```python
from build123d import *

# Parameters (mm, degrees)
SKETCH_8_R          = 1.5
SKETCH_8_W          = 15
SKETCH_8_H          = 16
EXTRUDE_4_DEPTH     = 4
SKETCH_9_R          = 7.5
EXTRUDE_5_DEPTH     = 5
SKETCH_10_R         = 5
EXTRUDE_6_DEPTH     = 5
SKETCH_12_R         = 4.5
EXTRUDE_7_DEPTH     = 1.1
SKETCH_14_R         = 1.45
CUT_EXTRUDE_1_DEPTH = 24.070760716
SKETCH_15_R         = 5
EXTRUDE_8_DEPTH     = 2
FILLET_2_R          = 0.75
SKETCH_16_R         = 1.45
CUT_EXTRUDE_2_DEPTH = 25.426624818


with BuildPart() as part:
    # 草图8 → 凸台-拉伸4 (new body)
    # profile 1 of 3: a face of its own
    with BuildSketch(Plane(origin=(0, 0, 0), x_dir=(1, 0, 0), z_dir=(0, 1, 0))):
        with BuildLine():
            Line((-7.5, 8), (-7.5, -8))
            ThreePointArc((-7.5, -8), (-15.5, 0), (-7.5, 8))
        make_face()
        with Locations(Location((-11, 0, 0), (0, 0, 270))):
            Circle(SKETCH_8_R, mode=Mode.SUBTRACT)
    # profile 2 of 3: a face of its own
    with BuildSketch(Plane(origin=(0, 0, 0), x_dir=(1, 0, 0), z_dir=(0, 1, 0))):
        Rectangle(SKETCH_8_W, SKETCH_8_H)
    # profile 3 of 3: a face of its own
    with BuildSketch(Plane(origin=(0, 0, 0), x_dir=(1, 0, 0), z_dir=(0, 1, 0))):
        with BuildLine():
            Line((7.5, 8), (7.5, -8))
            ThreePointArc((7.5, -8), (15.5, 0), (7.5, 8))
        make_face()
        with Locations(Location((11, 0, 0), (0, 0, 270))):
            Circle(SKETCH_8_R, mode=Mode.SUBTRACT)
    extrude(amount=EXTRUDE_4_DEPTH)

    # 草图9 → 凸台-拉伸5 (add)
    with BuildSketch(Plane(origin=(0, 4, 0), x_dir=(1, 0, 0), z_dir=(0, 1, 0))):
        with Locations(Location((0, 0, 0), (0, 0, 270))):
            Circle(SKETCH_9_R)
    extrude(amount=EXTRUDE_5_DEPTH)

    # 草图10 → 凸台-拉伸6 (add)
    with BuildSketch(Plane(origin=(0, 9, 0), x_dir=(1, 0, 0), z_dir=(0, 1, 0))):
        with Locations(Location((0, 0, 0), (0, 0, 270))):
            Circle(SKETCH_10_R)
    extrude(amount=EXTRUDE_6_DEPTH)

    # 草图12 → 凸台-拉伸7 (add)
    with BuildSketch(Plane(origin=(0, 14, 0), x_dir=(1, 0, 0), z_dir=(0, 1, 0))):
        with Locations(Location((0, 0, 0), (0, 0, 270))):
            Circle(SKETCH_12_R)
    extrude(amount=EXTRUDE_7_DEPTH)

    # 草图14 → 切除-拉伸1 (cut, through all)
    with BuildSketch(Plane.XZ):
        with Locations(Location((0, 0, 0), (0, 0, 270))):
            Circle(SKETCH_14_R)
    extrude(amount=-CUT_EXTRUDE_1_DEPTH, mode=Mode.SUBTRACT)

    # 草图15 → 凸台-拉伸8 (add)
    with BuildSketch(Plane(origin=(0, 15.1, 0), x_dir=(1, 0, 0), z_dir=(0, 1, 0))):
        with Locations(Location((0, 0, 0), (0, 0, 270))):
            Circle(SKETCH_15_R)
    extrude(amount=EXTRUDE_8_DEPTH)

    # 圆角2
    fillet_2_edges = [part.edges().sort_by_distance(p)[0] for p in [
        (0, 9, -7.5),
        (0, 17.1, -5),
    ]]
    fillet(fillet_2_edges, radius=FILLET_2_R)

    # 草图16 → 切除-拉伸2 (cut, through all)
    with BuildSketch(Plane(origin=(0, 0, 0), x_dir=(-1, 0, 0), z_dir=(0, -1, 0))):
        with Locations(Location((0, 0, 0), (0, 0, 90))):
            Circle(SKETCH_16_R)
    extrude(amount=-CUT_EXTRUDE_2_DEPTH, mode=Mode.SUBTRACT)


solid = part.part
```
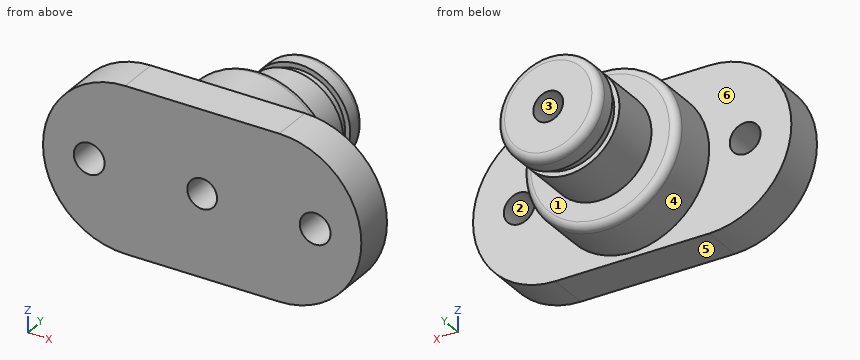
CAD build for the part. Positions are in the model's coordinates, mm. Face numbers are marked on the shaded views. A direction names the side the tool comes from. Coordinates: 2 decimals unless noted, no trailing zeros. Write each loop counter-clockwise with the first axis right and the second up, starting at its lowest first coordinate (ties: lowest second). Pieces come first, ordered by that corner, then holes. Notation, with made-up numbers: (2, 4) -> (36, 4) arc R21 ccw to (36, 25) -> close; hole circle Ø8 at (56, 27). An arc over 180 degrees is marked (long way). Return JSON: item names as keys, results as strings. Group by question number.
Q1. Pull direction Z, two halves, no side cores. Call the marked faces 1, 2, 3 and 4: released by +Z, released by -Z, zero draft, split by the parting line, or undercut.
Q2. Which spindle directions (+Z, -Z, +X, -X, +Y, -Y) get a long thin tool onto all of the face, cutting with end or side? Do the marked faces 5 and 6. Say none if no direction does.
Q3. Cut at B-B, the plane y = 10.5. Give the cut face in (x, z), then the cut area to 3 significant figures.
Q4. Cut at D-D, the plane x = 11.5. Give the cut face in (y, z).
Q5. Cut at A-A, the plane x = 0. Give the cut face in (y, z), then the cut area to 3 significant figures.
Q6. Drill centre lines: line 1 (X direction, y = 1.9, z = 0); line 2 (X direction, y = 5.5, z = 0); line 3 (X direction, y = 10.5, z = 0). Where is each one in solid material? Low to high.
Q7. Flat gauge pins, fed straight in: pin 1 (5 mm diameter, centred on x = 8, y = 8.5, fed in from -Z); pin 2 (1 mm diameter, centred on y = 3.5, z = -3, fed in from +X); pin 3 (2 mm diameter, centred on y = 7.5, z = -4.5, fed in from -X). Where does each tip first touch, or does it go through?
Q8. Cut at C-C, the plane z = 0. State how many separate pieces and enclosed holes the cut face has, then the cut area to 3 significant figures.
Returned:
{
 "1": {"face 1": "zero draft", "face 2": "undercut", "face 3": "undercut", "face 4": "split by the parting line"},
 "2": {"face 5": "-Z, +X, -X, +Y, -Y", "face 6": "+Y"},
 "3": {"outline": "circle Ø10 at (0, 0); hole circle Ø2.9 at (0, 0)", "area": "71.9 mm2"},
 "4": {"outline": "(0, -6.93) -> (4, -6.93) -> (4, -1.41) -> (0, -1.41) -> close; (0, 1.41) -> (4, 1.41) -> (4, 6.93) -> (0, 6.93) -> close"},
 "5": {"outline": "(0, -8) -> (4, -8) -> (4, -7.5) -> (8.25, -7.5) arc R0.75 ccw to (9, -6.75) -> (9, -5) -> (14, -5) -> (14, -4.5) -> (15.1, -4.5) -> (15.1, -5) -> (16.35, -5) arc R0.75 ccw to (17.1, -4.25) -> (17.1, -1.45) -> (0, -1.45) -> close; (0, 1.45) -> (17.1, 1.45) -> (17.1, 4.25) arc R0.75 ccw to (16.35, 5) -> (15.1, 5) -> (15.1, 4.5) -> (14, 4.5) -> (14, 5) -> (9, 5) -> (9, 6.75) arc R0.75 ccw to (8.25, 7.5) -> (4, 7.5) -> (4, 8) -> (0, 8) -> close", "area": "169 mm2"},
 "6": {"line 1": "x = -15.5 to -12.5, -9.5 to -1.45, 1.45 to 9.5, 12.5 to 15.5", "line 2": "x = -7.5 to -1.45, 1.45 to 7.5", "line 3": "x = -5 to -1.45, 1.45 to 5"},
 "7": {"pin 1": "stops at z = -5.09", "pin 2": "stops at x = 15.1", "pin 3": "stops at x = -6.63"},
 "8": {"separate pieces": "4", "enclosed holes": "0", "area": "205 mm2"}
}
